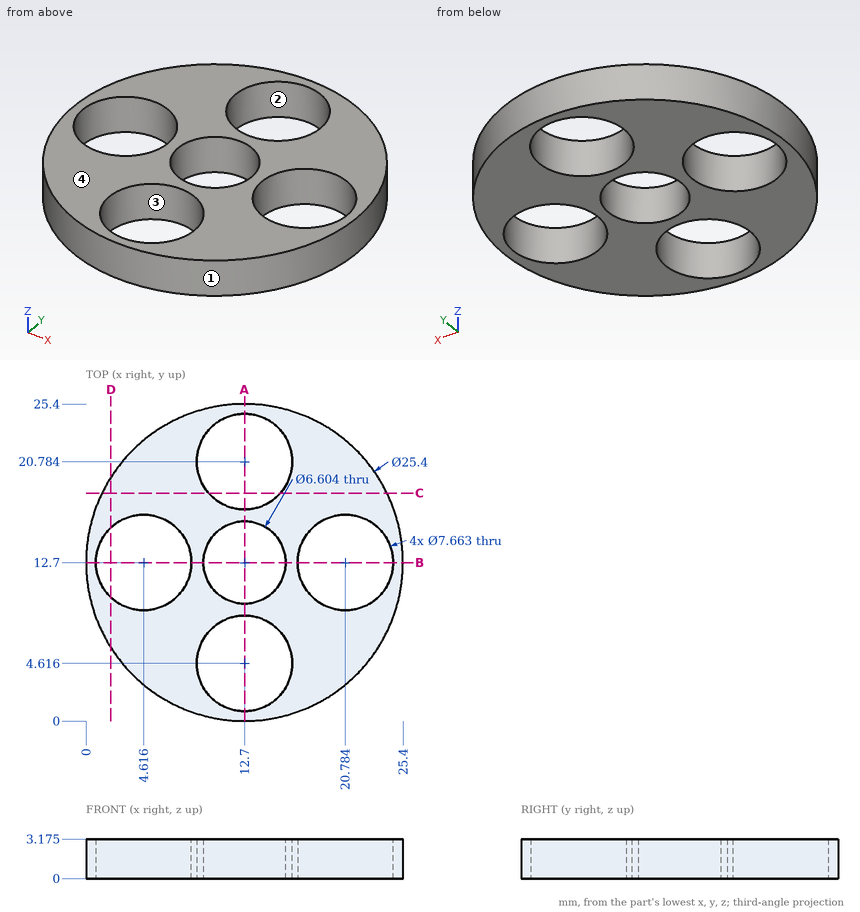
Verification items for this drawing (mm, ordinates from the low corner). Coordinates: 2 decimals unless noted, no trailing zeros. Order: outer loops, then holes, each group sorted by start corner. A loop starts at its lowest first (then second) coordinate and runs counter-clockwise, first axis right, second up. Notation, with made-up numbers: (66, 55) - (73, 55) arc R27 cw to (73, 74) - close; hole circle Ø8 at (76, -36). An arc over 180 degrees is marked (long way). Use one line per item in the form item = value.
1. Gauge pin test, flat end, axial feed: pin 1 (9 mm diameter, centred on x = 12.7, y = 20.78, fed in from +Z) (3 decimals). Record the tip position at first contact, or that the pin passes through.
Here are the results:
pin_1 = 3.175
2. Draft check along Y on the marked faces 1, 2, 3 and 4. Enter one of: pulls with the +Y half, pulls with the -Y half, needs draft (parallel to the pull), parting line crosses it, or undercut.
Here are the results:
face_1 = parting line crosses it
face_2 = undercut
face_3 = undercut
face_4 = needs draft
3. Section check D-D (x = 2). Record the boundary of the cut face in (y, z) (1 decimal).
Here are the results:
outline = (5.9, 0) - (9.9, 0) - (9.9, 3.2) - (5.9, 3.2) - close; (15.5, 0) - (19.5, 0) - (19.5, 3.2) - (15.5, 3.2) - close
4. Section check C-C (y = 18.25). Record the boundary of the cut face in (x, z) (1 decimal), then the cut area to 3 significant figures.
Here are the results:
outline = (1.3, 0) - (9.8, 0) - (9.8, 3.2) - (1.3, 3.2) - close; (15.6, 0) - (24.1, 0) - (24.1, 3.2) - (15.6, 3.2) - close
area = 54.3 mm²
5. Section check A-A (x = 12.7). Record the boundary of the cut face in (y, z) (1 decimal).
Here are the results:
outline = (0, 0) - (0.8, 0) - (0.8, 3.2) - (0, 3.2) - close; (8.4, 0) - (9.4, 0) - (9.4, 3.2) - (8.4, 3.2) - close; (16, 0) - (17, 0) - (17, 3.2) - (16, 3.2) - close; (24.6, 0) - (25.4, 0) - (25.4, 3.2) - (24.6, 3.2) - close
6. Scan lines: line 1 (Y direction, x = 12.7, z = 1.3); line 2 (X direction, y = 11.5, z = 2.35) (1 decimal); line 3 (Y direction, x = 22.5, z = 2.15) (1 decimal). Record each from-to range of solid material in increasing order.
Here are the results:
line_1 = 0 to 0.78, 8.45 to 9.4, 16 to 16.95, 24.62 to 25.4
line_2 = 0.1 to 1, 8.3 to 9.6, 15.8 to 17.1, 24.4 to 25.3
line_3 = 4.6 to 9.3, 16.1 to 20.8
